Could you check a few things on this model? Use its own coordinates, in mm. Face numbers are marked on the shaded views. A direction names the side the tool comes from. Coordinates: 2 decimals unless noted, no trailing zeros. Write each loop counter-clockwise with the first axis right and the second up, starting at its lowest first coordinate (ties: lowest second). Pieces come first, ordered by that corner, then holes.
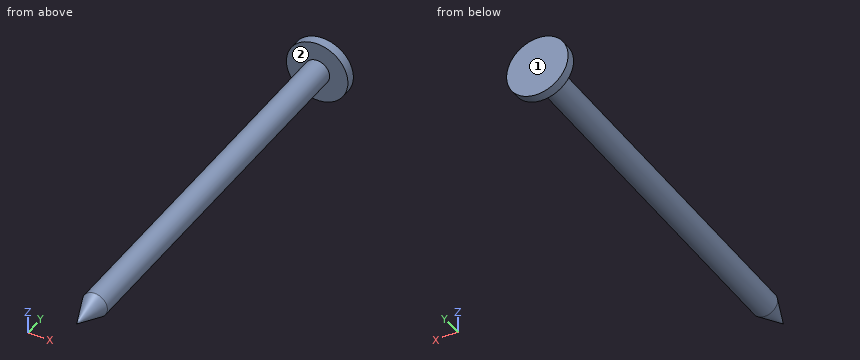
```python
from build123d import *

# Parameters (mm, degrees)
SKETCH1_R           = 0.6
BOSS_EXTRUDE1_DEPTH = 18.25
SKETCH2_R           = 1.475
BOSS_EXTRUDE2_DEPTH = 0.45


with BuildPart() as part:
    # Sketch1 → Boss-Extrude1 (new body)
    with BuildSketch(Plane(origin=(0, 0, 0), x_dir=(1, 0, 0), z_dir=(0, 1, 0))):
        with Locations(Location((0, 0, 0), (0, 0, 270))):
            Circle(SKETCH1_R)
    extrude(amount=BOSS_EXTRUDE1_DEPTH)

    # Sketch2 → Boss-Extrude2 (add)
    with BuildSketch(Plane(origin=(0, 18.25, 0), x_dir=(1, 0, 0), z_dir=(0, 1, 0))):
        with Locations(Location((0, 0, 0), (0, 0, 270))):
            Circle(SKETCH2_R)
    extrude(amount=BOSS_EXTRUDE2_DEPTH)

    # Sketch4 → Revolve1 (revolve)
    with BuildSketch(Plane(origin=(0, 0, 0), x_dir=(0, 0, -1), z_dir=(1, 0, 0)), mode=Mode.PRIVATE) as revolve1_sk:
        Polygon((0, 0), (0, -1.5), (0.6, 0), align=None)
    revolve(revolve1_sk.sketch.rotate(Axis((0, 0, 0), (0, -1, 0)), 180), axis=Axis((0, 0, 0), (0, -1, 0)))


solid = part.part
```
Item 1: Which directions (+Z, -Z, +X, -X, +Y, -Y) give clear straight access to the entire face, cutting with the end or side of a thin tool? Please do the marked faces 1 and 2.
Item 2: Will these pins go through, and if not, where does the flat tip stop? pin 1 Ø1.5 at (x, y) = (-0.5, 15.5) entering from -Z; pin 2 Ø1.5 at (x, y) = (0, 2) entering from +Z.
Item 3: I want a section at C-C, the plane z = -0.95. List the corners of the cut face in (x, y) for me.
Item 4: I want a section at B-B, the plane x = -0.85. List the corners of the cut face in (y, z) for me.
Item 5: If I drill on line 1 along Y through (x, z) = (-1.1, -0.65); line 2 along X through (y, z) = (9.5, 0); line 3 along Z through (x, y) = (0.45, 10.75), over which ranges is the centre line in solid material (lowest first)?
Item 6: I want a section at A-A, the plane y = 2. List the corners of the cut face in (x, z) for me, then the cut area to 3 significant figures.
Taken from the geometry:
1. face 1: +Z, -Z, +X, -X, +Y
1. face 2: -Y
2. pin 1: stops at z = -0.6
2. pin 2: stops at z = 0.6
3. outline: (-1.13, 18.25) - (1.13, 18.25) - (1.13, 18.7) - (-1.13, 18.7) - close
4. outline: (18.25, -1.21) - (18.7, -1.21) - (18.7, 1.21) - (18.25, 1.21) - close
5. line 1: y = 18.25 to 18.7
5. line 2: x = -0.6 to 0.6
5. line 3: z = -0.4 to 0.4
6. outline: circle Ø1.2 at (0, 0)
6. area: 1.13 mm2
